For this review, take the finished solid that the model builds, in its own axes (mm). Face numbers are marked on the shaded views. A direction names the side the tool comes from. Round coordinates to 2 decimals unless told otherwise and drop trailing zeros. Write each loop counter-clockwise with the first axis right and the second up, starting at its lowest first coordinate (ties: lowest second). Pieces come first, ordered by that corner, then holes. Notation, with made-up numbers: (-0.5, -28.75) -> (41.5, -28.75) arc R12 cw to (41.5, -23.75) -> close; hole circle Ø5 at (-34.75, 56). An arc over 180 degrees is marked (long way). Write item = value, one per line. Start each with the question number.
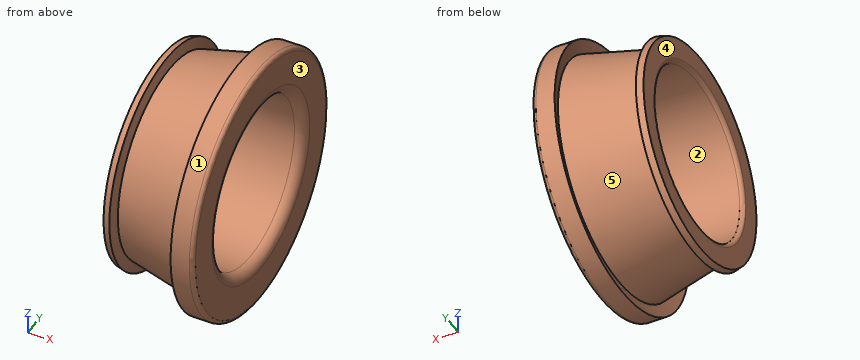
```python
from build123d import *


with BuildPart() as part:
    # Esquisse1 → Base-Révolution (revolve)
    with BuildSketch(Plane.XY, mode=Mode.PRIVATE) as base_r_volution_sk:
        with BuildLine():
            Line((0, 14), (0, 18.65))
            ThreePointArc((0, 18.65), (-0.175735931, 19.074264069), (-0.6, 19.25))
            Line((-0.6, 19.25), (-3.385649604, 19.25))
            Line((-3.385649604, 19.25), (-2.868011513, 17.318148347))
            Line((-2.868011513, 17.318148347), (-13.569257226, 14.798339466))
            Line((-13.569257226, 14.798339466), (-14, 16.405893383))
            Line((-14, 16.405893383), (-15, 16.137944191))
            Line((-15, 16.137944191), (-15, 13.1))
            ThreePointArc((-15, 13.1), (-14.824264069, 12.675735931), (-14.4, 12.5))
            Line((-14.4, 12.5), (-1.5, 12.5))
            ThreePointArc((-1.5, 12.5), (-0.439339828, 12.939339828), (0, 14))
        make_face()
    revolve(base_r_volution_sk.sketch.rotate(Axis((0, 0, 0), (-1, 0, 0)), 90), axis=Axis((0, 0, 0), (-1, 0, 0)))


solid = part.part
```
1. Consider section A-A, the plane y = 0. Give the boundary of the cut face in (x, z), then the cut area to 3 significant figures.
2. Draft analysis for pull direction Y (two halves, no side actions). For the marked faces 1, 2 and 3, state which applies: +Y half, -Y half, draft (parallel to the pull), parting line (faces both ways), or undercut.
3. Consider section C-C, the plane x = -7.5. Give the boundary of the cut face in (y, z), then the cut area to 3 significant figures.
4. Clearance check with flat-ended pins moving along their axes: pin 1 Ø1 at (x, y) = (-3.5, -3.5) entering from -Z; pin 2 Ø2 at (x, y) = (-5.5, -7.5) entering from -Z; pin 3 Ø5 at (x, y) = (-7, -9) entering from -Z; pin 4 Ø12 at (y, z) = (-6.5, 8) entering from -X. State where each tip first meets the part, or that it passes through.
5. Machinability: for the marked faces 4 and 5, which of the approach directions +Z, -Z, +X, -X, +Y, -Y give a long, thin tool a straight path to every point of the face, cutting with its end or side? Answer none if there is none.
6. Wall thickness on L1, parallel to Z at x = -1.5, y = 4; L2, parallel to Y at x = -9, z = 8; L3, parallel to Z at x = -10, y = -3: over which ranges is each line inside the solid? List them lowest first. Write a range as from..to.
Outcome:
q1.outline = (-15, -16.14) -> (-14, -16.41) -> (-13.57, -14.8) -> (-2.87, -17.32) -> (-3.39, -19.25) -> (-0.6, -19.25) arc R0.6 ccw to (0, -18.65) -> (0, -14) arc R1.5 ccw to (-1.5, -12.5) -> (-14.4, -12.5) arc R0.6 ccw to (-15, -13.1) -> close; (-15, 13.1) arc R0.6 ccw to (-14.4, 12.5) -> (-1.5, 12.5) arc R1.5 ccw to (0, 14) -> (0, 18.65) arc R0.6 ccw to (-0.6, 19.25) -> (-3.39, 19.25) -> (-2.87, 17.32) -> (-13.57, 14.8) -> (-14, 16.41) -> (-15, 16.14) -> close
q1.area = 125 mm2
q2.face_1 = parting line
q2.face_2 = undercut
q2.face_3 = draft
q3.outline = circle Ø32.45 at (0, 0); hole circle Ø25 at (0, 0)
q3.area = 336 mm2
q4.pin_1 = -19.01
q4.pin_2 = -15.45
q4.pin_3 = -15.17
q4.pin_4 = -15
q5.face_4 = +Z, -Z, -X, +Y, -Y
q5.face_5 = none
q6.L1 = -18.83..-11.84, 11.84..18.83
q6.L2 = -13.71..-9.6, 9.6..13.71
q6.L3 = -15.35..-12.13, 12.13..15.35
